Study the drawing (mm; zero at the part's minimum x, y, z) and answer. A direction names the side the tool comes from. Coordinates: 2 decimals unless noted, no trailing zeros. Loops run counter-clockwise (first coordinate to the right, second up) from the corner with the lowest first, then second, coordinate; pieces in that order, holes last. Notation, with made-up numbers: (49, 41) -> (72, 41) arc R4 cw to (72, 48) -> close; hole circle Ø10 at (54.5, 38). An arc over 180 degrees is marked (long way). Answer in a Markdown table with one row per item.
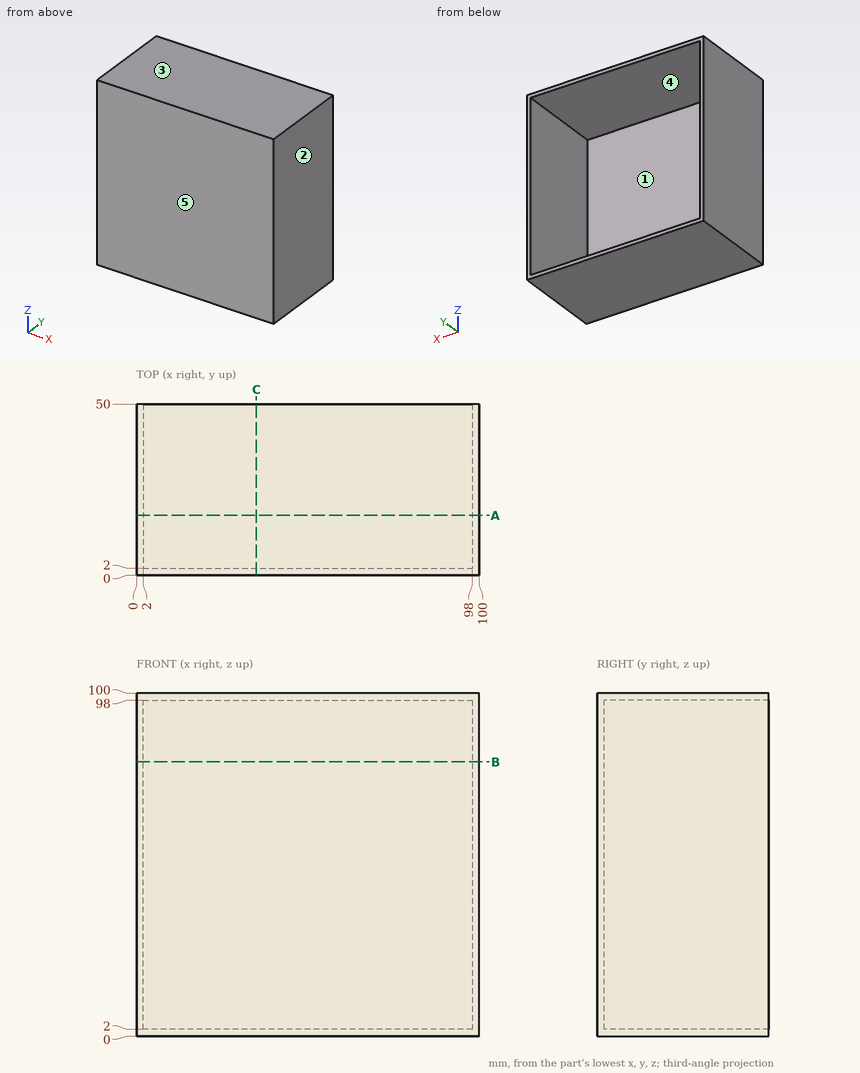
1. A cutting plane is placed at A-A on y = 17.5. Give the vertices of the cut face in (x, z), and give its area (3 significant figures).
A:
| item | result |
|---|---|
| outline | (0, 0) -> (100, 0) -> (100, 100) -> (0, 100) -> close; hole (2, 2) -> (98, 2) -> (98, 98) -> (2, 98) -> close |
| area | 784 mm2 |
2. A cutting plane is placed at C-C on x = 35. Give the vertices of the cut face in (y, z), and give its area (3 significant figures).
A:
| item | result |
|---|---|
| outline | (0, 0) -> (50, 0) -> (50, 2) -> (2, 2) -> (2, 98) -> (50, 98) -> (50, 100) -> (0, 100) -> close |
| area | 392 mm2 |
3. A tool of negligible diameter and unlimited length cuts with its end or side. For the marked faces 4 and 5, from which of +Z, -Z, +X, -X, +Y, -Y can it reach the whole face along a straight path? Write none if from no direction.
A:
| item | result |
|---|---|
| face 4 | +Y |
| face 5 | +Z, -Z, +X, -X, -Y |
4. A cutting plane is placed at B-B on z = 80. Give the vertices of the cut face in (x, y).
A:
| item | result |
|---|---|
| outline | (0, 0) -> (100, 0) -> (100, 50) -> (98, 50) -> (98, 2) -> (2, 2) -> (2, 50) -> (0, 50) -> close |
5. The mould has two halves that part along X. Classify the marked faces 1, 2 and 3: pulls with the +X half, pulls with the -X half, needs draft (parallel to the pull), parting line crosses it, or undercut.
A:
| item | result |
|---|---|
| face 1 | undercut |
| face 2 | pulls with the +X half |
| face 3 | needs draft |
6. Find the intervals of material crossed by probe 1 along Z at (x, y) = (54.5, 37.5); probe 2 along Y at (x, z) = (65, 74.5), in increasing order.
A:
| item | result |
|---|---|
| probe 1 | z = 0 to 2, 98 to 100 |
| probe 2 | y = 0 to 2 |
